Work out the finished part from the listing and answer in its coordinate system (mm). A direction names the side the tool comes from. Coordinates: 2 decimals unless noted, no trailing zeros. Write each loop counter-clockwise with the first axis right and the second up, starting at its lowest first coordinate (ties: lowest second). Pieces come first, ordered by that corner, then holes. Notation, with made-up numbers: (-29.5, 44.5) - (1.5, 44.5) arc R18 cw to (1.5, 68.5) - close; hole circle Ø6 at (41, 71). An arc over 180 degrees is marked (long way). Use one line per item in the form item = value. Start each with the question number.
Item 1: A cutting plane is placed at D-D (z = 6.25). Write down the section's boundary in (x, y), then the cut area to 3 significant figures.
Item 2: A cutting plane is placed at A-A (y = 12.25). Write down the section's boundary in (x, z).
Item 3: Determine the mould class of faces 1 (the flat face through (-8, 16, 14)), 2 (the flat face through (14, -1.38, 7)), 3 (the cylindrical face through (13, -2.39, 3.55)) for opening direction Z: released by +Z, released by -Z, zero draft, split by the parting line, or undercut.
Item 4: For faces 4 (the flat face through (-31, -1.38, 7)), 5 (the flat face through (8.93, 6, 7)), 6 (the flat face through (11.93, 8, 7)), determine the directions among +Z, -Z, +X, -X, +Y, -Y from which every point of the face is accessible in a straight line to the end or side of a thin tool.
Item 5: Consider probe 1 along Z at (x, y) = (14.43, -1.95); probe 2 along X at (y, z) = (14.75, 2.5); probe 3 along X at (y, z) = (-2.25, 4). Determine where each line is inside the solid, lowest interval first.
Item 6: A cutting plane is placed at C-C (z = 4). Write down the section's boundary in (x, y).
Item 7: Given pin 1 (1.5 mm diameter, centred on x = -30.5, z = 4, fed in from +Y); pin 2 (1.5 mm diameter, centred on x = -7.5, y = 15, fed in from +Z); pin 3 (2.5 mm diameter, centred on x = 13.5, z = 6, fed in from +Y); pin 4 (7 mm diameter, centred on y = 8, z = 4, fed in from +X), each flat-ended and moving along its own axis, determine where each tip first touches the part or whether it passes through.
Item 8: A cutting plane is placed at B-B (x = -31.17). Write down the section's boundary in (y, z).
from build123d import *

# Parameters (mm, degrees)
BOSS_EXTRUDE1_DEPTH      = 14
F_3_0_3_DIAMETER_HOLE1_D = 3


with BuildPart() as part:
    # Sketch2 → Boss-Extrude1 (new body)
    with BuildSketch(Plane.XY):
        Polygon((11.93, -3.38), (16.93, -3.38), (16.93, -1.38), (11.93, -1.38), (11.93, 18.62), (-28.67, 18.62), (-28.67, -1.38), (-33.67, -1.38), (-33.67, -3.38), (-12.23, -3.38), (-25.67, -3.38), (-25.67, 15.62), (8.93, 15.62), (8.93, -3.38), align=None)
    extrude(amount=BOSS_EXTRUDE1_DEPTH)

    # Ø3.0 (3) Diameter Hole1 (through all)
    with Locations(Plane(origin=(0, -1.38, 0), x_dir=(1, 0, 0), z_dir=(0, 1, 0))):
        with Locations((14.43, -4), (-31.17, -4)):
            Hole(F_3_0_3_DIAMETER_HOLE1_D / 2)


solid = part.part
Answer:
q1.outline = (-33.67, -3.38) - (-25.67, -3.38) - (-25.67, 15.62) - (8.93, 15.62) - (8.93, -3.38) - (16.93, -3.38) - (16.93, -1.38) - (11.93, -1.38) - (11.93, 18.62) - (-28.67, 18.62) - (-28.67, -1.38) - (-33.67, -1.38) - close
q1.area = 256 mm²
q2.outline = (-28.67, 0) - (-25.67, 0) - (-25.67, 14) - (-28.67, 14) - close; (8.93, 0) - (11.93, 0) - (11.93, 14) - (8.93, 14) - close
q3.face_1 = released by +Z
q3.face_2 = zero draft
q3.face_3 = undercut
q4.face_4 = +Z, -Z, -X, +Y
q4.face_5 = +Z, -Z, -Y
q4.face_6 = +Z, -Z, +X, +Y
q5.probe_1 = 0 to 2.5, 5.5 to 14
q5.probe_2 = -28.67 to -25.67, 8.93 to 11.93
q5.probe_3 = -33.67 to -32.67, -29.67 to -25.67, 8.93 to 12.93, 15.93 to 16.93
q6.outline = (-33.67, -3.38) - (-32.67, -3.38) - (-32.67, -1.38) - (-33.67, -1.38) - close; (-29.67, -3.38) - (-25.67, -3.38) - (-25.67, 15.62) - (8.93, 15.62) - (8.93, -3.38) - (12.93, -3.38) - (12.93, -1.38) - (11.93, -1.38) - (11.93, 18.62) - (-28.67, 18.62) - (-28.67, -1.38) - (-29.67, -1.38) - close; (15.93, -3.38) - (16.93, -3.38) - (16.93, -1.38) - (15.93, -1.38) - close
q7.pin_1 = through
q7.pin_2 = 14
q7.pin_3 = -1.38
q7.pin_4 = 11.93
q8.outline = (-3.38, 0) - (-1.38, 0) - (-1.38, 2.5) - (-3.38, 2.5) - close; (-3.38, 5.5) - (-1.38, 5.5) - (-1.38, 14) - (-3.38, 14) - close
